Here's the drawing with two shaded views (mm, measured from the low corner). I have some questions. A direction names the side the tool comes from. Give positions to 0.01 mm unless a question says otherwise; leave off trailing zeros. Loops run counter-clockwise (first coordinate to the right, second up) from the corner with the lowest first, then second, coordinate; pieces in that order, holes last. Notation, with made-up numbers: M 50.25,28 L 66.25,28 A16 cw 66.25,37 Z; hole C -21,-8 d6. An arc over 180 degrees is marked long. Answer in a Markdown table with one row per item. Add a question column.
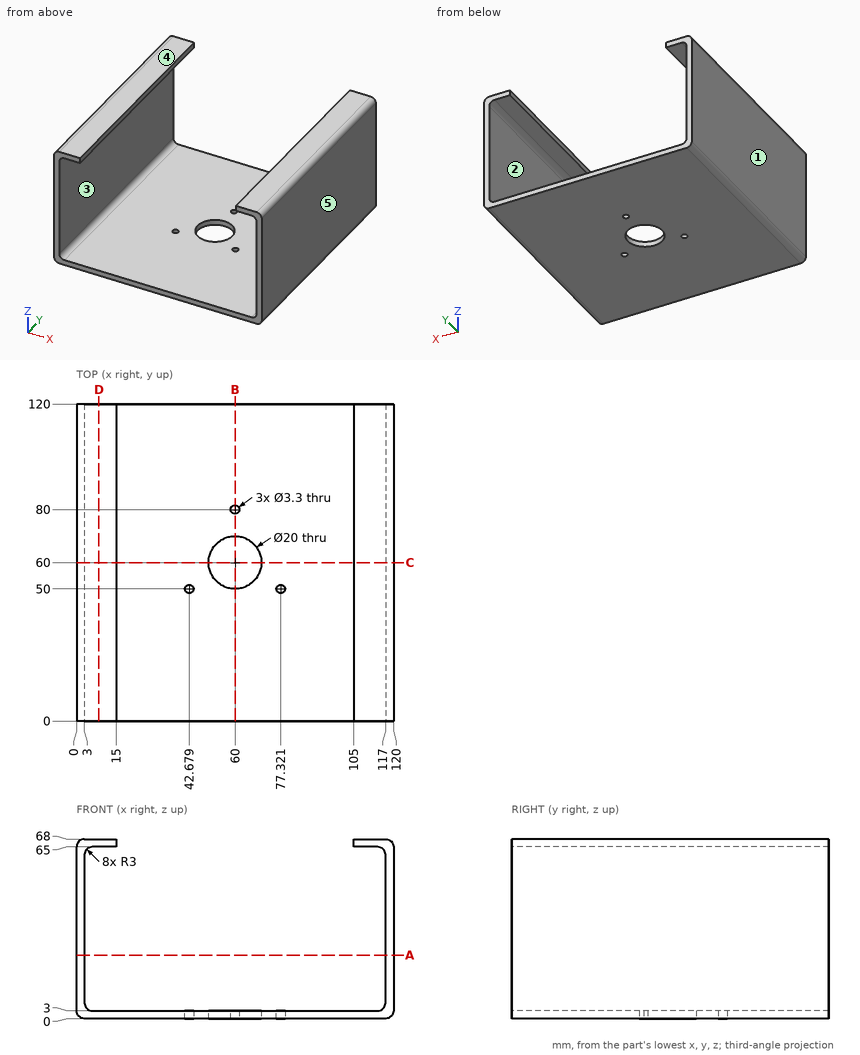
Item 1: If we mould it in two halves opening along X, with no side actions, what happens to the marked faces 3, 4 and 5? For each: +X half, -X half, draft (parallel to the pull), parting line (faces both ways), or undercut.
Item 2: I need wall thicknesses on L1, parallel to Z at x = 6, y = 96; L2, parallel to X at y = 98.5, z = 10; L3, parallel to Y at x = 60, z = 2.1. Which ranges of each line are inside material? Lowest first, please.
Item 3: Suppose I cut it at B-B (x = 60). List the corners of the cut face in (y, z) for me, then the cut area to 3 significant figures.
Item 4: Suppose I cut it at D-D (x = 8.5). List the corners of the cut face in (y, z) for me, then the cut area to 3 significant figures.
Item 5: For P1, Ø2.5, axis at y = 90, z = 66.5, coming from the -X side; P2, Ø1.5, axis at y = 40, z = 67, coming from the +X side; P3, Ø1, axis at x = 70.5, y = 98, coming from the +Z side, each with a flat end and sliding along its axis, tell me the tip position at first contact or that it passes through.
Item 6: For the marked faces 1 and 2, which set-ups out of +Z, -Z, +X, -X, +Y, -Y let a thin tool reach every point of the face, with its end or its side?
Item 7: Suppose I cut it at C-C (y = 60). List the corners of the cut face in (x, z) for me.
Item 8: Suppose I cut it at A-A (z = 24). List the corners of the cut face in (x, y) for me.
Values found:
| question | item | result |
|---|---|---|
| 1 | face 3 | undercut |
| 1 | face 4 | draft |
| 1 | face 5 | +X half |
| 2 | L1 | 0 to 3, 65 to 68 |
| 2 | L2 | 0 to 3, 117 to 120 |
| 2 | L3 | 0 to 50, 70 to 78.35, 81.65 to 120 |
| 3 | outline | M 0,0 L 50,0 L 50,3 L 0,3 Z; M 70,0 L 78.35,0 L 78.35,3 L 70,3 Z; M 81.65,0 L 120,0 L 120,3 L 81.65,3 Z |
| 3 | area | 290 mm² |
| 4 | outline | M 0,0 L 120,0 L 120,3 L 0,3 Z; M 0,65 L 120,65 L 120,68 L 0,68 Z |
| 4 | area | 720 mm² |
| 5 | P1 | x = 0.01 |
| 5 | P2 | x = 119.73 |
| 5 | P3 | z = 3 |
| 6 | face 1 | +Z, -Z, -X, +Y, -Y |
| 6 | face 2 | +Y, -Y |
| 7 | outline | M 0,3 A3 ccw 3,0 L 50,0 L 50,3 L 6,3 A3 cw 3,6 L 3,62 A3 cw 6,65 L 15,65 L 15,68 L 3,68 A3 ccw 0,65 Z; M 70,0 L 117,0 A3 ccw 120,3 L 120,65 A3 ccw 117,68 L 105,68 L 105,65 L 114,65 A3 cw 117,62 L 117,6 A3 cw 114,3 L 70,3 Z |
| 8 | outline | M 0,0 L 3,0 L 3,120 L 0,120 Z; M 117,0 L 120,0 L 120,120 L 117,120 Z |
